from build123d import *

# Parameters (mm, degrees)
F1_DEPTH     = 63.5
F0_W         = 25.4
F0_H         = 19.05
F2_DEPTH     = 25.4
F3_DEPTH     = 7.9375
F5_R         = 5.08
F6_T         = 5.08
F6_T3_DEPTH  = 29.21
F6_T5_DEPTH  = 27.6225
F6_T7_DEPTH  = 73.66
F6_T9_DEPTH  = 27.6352
F6_T11_DEPTH = 27.6225
F6_T14_ANGLE = 84.6365269518
F6_T16_ANGLE = 180.000000001
F6_T18_ANGLE = 180.000000001
F6_T20_ANGLE = 84.6365269518


# Not quite as in the source:
# - a shell that OpenCascade refuses in one call is made with other operations: the cavity is built on its own and cut out


with BuildPart() as f1:
    # F0 (on Front) → F1 (new body, symmetric)
    with BuildSketch(Plane.XZ):
        Polygon((22.225, 9.525), (-41.275, 9.525), (-41.275, -9.525), (41.275, -9.525), (41.275, 9.525), align=None)
    extrude(amount=F1_DEPTH, both=True)

    # F0 (on Front) → F2 (join, symmetric)
    with BuildSketch(Plane.XZ):
        with BuildLine():
            Line((22.225, 27.0002), (22.225, 9.525))
            Line((22.225, 9.525), (41.275, 9.525))
            Line((41.275, 9.525), (41.275, 27.0002))
            ThreePointArc((41.275, 27.0002), (45.9246798487, 38.2255201513), (57.15, 42.8752))
            Line((57.15, 42.8752), (60.325, 42.8752))
            Line((60.325, 42.8752), (60.325, 61.9252))
            Line((60.325, 61.9252), (57.15, 61.9252))
            add(Edge.make_bspline(
                [(53.8854342407, 61.7722898912), (54.9842067368, 61.8365871986), (56.0728453275, 61.8876096574), (57.15, 61.9252)],
                knots=[108.5245810491, 108.5245810491, 108.5245810491, 108.5245810491, 111.5045361635, 111.5045361635, 111.5045361635, 111.5045361635], degree=3))
            ThreePointArc((53.8854342407, 61.7722898912), (31.3258777096, 50.5133948686), (22.225, 27.0002))
        make_face()
        with Locations((73.025, 52.4002)):
            Rectangle(F0_W, F0_H)
    extrude(amount=F2_DEPTH, both=True)

    # F0 (on Front) → F3 (join, symmetric)
    with BuildSketch(Plane.XZ):
        with BuildLine():
            add(Edge.make_bspline(
                [(-41.275, 9.525), (-39.5856284224, 39.4828766469), (13.870125209, 59.4306981306), (53.8854342407, 61.7722898912)],
                knots=[0, 0, 0, 0, 108.5245810491, 108.5245810491, 108.5245810491, 108.5245810491], degree=3))
            Line((-41.275, 9.525), (22.225, 9.525))
            Line((22.225, 9.525), (22.225, 27.0002))
            ThreePointArc((22.225, 27.0002), (31.3258777096, 50.5133948686), (53.8854342407, 61.7722898912))
        make_face()
    extrude(amount=F3_DEPTH, both=True)

    # F0 (on Front) → F4 (revolve)
    with BuildSketch(Plane.XZ):
        Polygon((85.725, 66.675), (85.725, 61.9252), (85.725, 42.8752), (85.725, 38.1), (111.125, 38.1), (111.125, 66.675), align=None)
    revolve(axis=Axis((85.725, 0, 52.3875), (0, 0, 1)))

    # F5
    f5_edges = [f1.edges().sort_by_distance(p)[0] for p in [
        (41.275, -63.5, 0),
        (-41.275, -63.5, 0),
        (41.275, 63.5, 0),
        (-41.275, 63.5, 0),
    ]]
    fillet(f5_edges, radius=F5_R)

    # F6: shell of thickness 5.08, made by hand


with BuildPart() as f6_core1:
    # F6_t2: copy of F1
    add(f1.part)

    # the walls: a layer under each face that stays
    f6_faces = [f6_core1.faces().sort_by_distance(p)[0] for p in [
        (0, 35.71875, 9.525),
        (41.275, 0, 8.7376),
        (32.8083333333, 25.4, 18.2583666667),
        (0, 63.5, 0),
        (22.225, 16.66875, 18.2626),
        (6.3052171204, 7.9375, 35.6486449456),
        (-41.275, 0, 0),
        (45.9246798487, 0, 38.2255201513),
        (32.8083333333, -25.4, 18.2583666667),
        (0, -35.71875, 9.525),
        (31.3258777096, 16.66875, 50.5133948686),
        (61.9125, 16.9333333333, 42.8752),
        (98.425, 21.9970452561, 42.8625),
        (61.9125, 16.9333333333, 61.9252),
        (55.5258238042, 12.7, 61.8587600574),
        (-8.0670094249, 3.96875, 46.0047517779),
        (-8.0670094249, -3.96875, 46.0047517779),
        (0, -63.5, 0),
        (31.3258777096, -16.66875, 50.5133948686),
        (22.225, -16.66875, 18.2626),
        (55.5258238042, -12.7, 61.8587600574),
        (6.3052171204, -7.9375, 35.6486449456),
        (85.725, 0, 66.675),
    ]]
    thicken(f6_faces, amount=-F6_T, mode=Mode.SUBTRACT)

    # F6_s4 → F6_t3 (cut)
    with BuildSketch(Plane.YZ.offset(17.145)):
        Polygon((25.4508, 9.5758), (25.4, 4.445), (20.32, 4.445), (20.32, 9.525), align=None)
        Polygon((-25.4508, 9.5758), (-20.32, 9.525), (-20.32, 4.445), (-25.4, 4.445), align=None)
    extrude(amount=F6_T3_DEPTH, mode=Mode.SUBTRACT)

    # F6_s6 → F6_t5 (cut)
    with BuildSketch(Plane.XZ.offset(-30.48)):
        Polygon((22.1742, 9.5758), (22.225, 4.445), (27.305, 4.445), (27.305, 9.525), align=None)
    extrude(amount=F6_T5_DEPTH, mode=Mode.SUBTRACT)

    # F6_s8 → F6_t7 (cut)
    with BuildSketch(Plane.YZ.offset(-46.355)):
        Polygon((7.9883, 9.5758), (7.9375, 4.445), (2.8575, 4.445), (2.8575, 9.525), align=None)
        Polygon((-7.9883, 9.5758), (-7.9375, 4.445), (-2.8575, 4.445), (-2.8575, 9.525), align=None)
    extrude(amount=F6_T7_DEPTH, mode=Mode.SUBTRACT)

    # F6_s10 → F6_t9 (cut)
    with BuildSketch(Plane.XY.offset(4.445)):
        Polygon((22.1742, 7.9883), (27.305, 7.9375), (27.305, 2.8575), (22.225, 2.8575), align=None)
        Polygon((22.1742, -7.9883), (27.305, -7.9375), (27.305, -2.8575), (22.225, -2.8575), align=None)
    extrude(amount=F6_T9_DEPTH, mode=Mode.SUBTRACT)

    # F6_s12 → F6_t11 (cut)
    with BuildSketch(Plane.XZ.offset(2.8575)):
        Polygon((22.1742, 9.5758), (22.225, 4.445), (27.305, 4.445), (27.305, 9.525), align=None)
    extrude(amount=F6_T11_DEPTH, mode=Mode.SUBTRACT)

    # F6_s13 → F6_t14 (revolve, cut)
    with BuildSketch(Plane.XY.offset(27.0002)):
        Polygon((22.1742, 7.9883), (22.225, 2.8575), (27.305, 2.8575), (27.305, 7.9375), align=None)
    revolve(axis=Axis((57.15, 7.9375, 27.0002), (0, 1, 0)), revolution_arc=F6_T14_ANGLE, mode=Mode.SUBTRACT)

    # F6_s15 → F6_t16 (revolve, cut)
    with BuildSketch(Plane.YZ.offset(85.725)):
        Polygon((25.4508, 42.8244), (25.4, 47.9552), (20.32, 47.9552), (20.32, 42.8752), align=None)
    revolve(axis=Axis((85.725, 0, 42.8752), (0, 0, 1)), revolution_arc=F6_T16_ANGLE, mode=Mode.SUBTRACT)

    # F6_s17 → F6_t18 (revolve, cut)
    with BuildSketch(Plane.YZ.offset(85.725)):
        Polygon((25.4508, 61.976), (20.32, 61.9252), (20.32, 56.8452), (25.4, 56.8452), align=None)
    revolve(axis=Axis((85.725, 0, 61.9252), (0, 0, 1)), revolution_arc=F6_T18_ANGLE, mode=Mode.SUBTRACT)

    # F6_s19 → F6_t20 (revolve, cut)
    with BuildSketch(Plane.XY.offset(27.0002)):
        Polygon((22.1742, -7.9883), (27.305, -7.9375), (27.305, -2.8575), (22.225, -2.8575), align=None)
    revolve(axis=Axis((57.15, -7.9375, 27.0002), (0, 1, 0)), revolution_arc=F6_T20_ANGLE, mode=Mode.SUBTRACT)


with BuildPart() as f1_1:
    add(f1.part)

    # what is left inside the walls is the cavity
    f6_cavity = [f6_core1.part.solids().sort_by_distance(p)[0] for p in [
        (0, 19.473333, -9.4742),
    ]]
    add(f6_cavity, mode=Mode.SUBTRACT)


solid = f1_1.part
Here's how the part is built. I have some questions about the finished solid (model axes, mm). A direction names the side the tool comes from. Give positions to 0.01 mm unless a question says otherwise; leave off trailing zeros. Order: outer loops, then holes, each group sorted by start corner. A loop starts at its lowest first (then second) coordinate and runs counter-clockwise, first axis right, second up. Notation, with made-up numbers: M -38.5,65.25 L 19.5,65.25 A16 cw 19.5,88.25 Z; hole C 37,51 d1. An arc over 180 degrees is marked long. Answer as a JSON object with one key per item and string values. Group by question number.
1) Please list where these lines run through material, in increasing order: L1, parallel to Y at x = 36, z = 46; L2, parallel to Y at x = 10, z = -5.5; L3, parallel to X at y = 0, z = 44 (3 decimals). Write a range as [from, to].
2) On a 3-axis mill with a long thin cutter (end or side, diameter ignored), from which of +Z, -Z, +X, -X, +Y, -Y can I reach the whole of each face in a straight line? I mean faces 5 (the flat face through (60, -2, 61.925)), 6 (the flat face through (27.305, -12, 16)), 7 (the flat face through (65, 0, 56.845)). Say none if no direction works.
3) Suppose I cut it at A-A, the plane z = 6.5. Write out the boundary of the cut face in (x, y) (1 decimal), plus the area to 3 significant figures.
4) We'd pull the mould along X, two halves only. Please class faces 1 (the cylindrical face through (39.8, -62, 0.1)), 2 (the flat face through (-41.275, -1, 0)), 3 (the flat face through (47.7, 20.32, 46.3)), 4 (the flat face through (-2, 2.858, 24)): pulls with the +X half, pulls with the -X half, needs draft (parallel to the pull), parting line crosses it, or undercut.
5) I'm going to push flat-ended pins straight in: pin 1 Ø8.5 at (y, z) = (14, 12) entering from +X (3 decimals); pin 2 Ø8 at (x, z) = (25.5, 26.5) entering from +Y; pin 3 Ø15 at (x, y) = (73.5, 9) entering from -Z. Where does each tip first touch, or does it pass through?
6) Suppose I cut it at B-B, the plane y = 55. Write out the boundary of the cut face in (x, z) (3 decimals), plus the area to 3 significant figures.
Results found:
{
 "1": {"L1": "[-25.4, -20.32], [20.32, 25.4]", "L2": "[-63.5, -58.42], [58.42, 63.5]", "L3": "[-12.006, -0.213], [44.898, 65.405], [106.045, 111.125]"},
 "2": {"face 5": "+Z, -X", "face 6": "-Z", "face 7": "none"},
 "3": {"outline": "M -41.3,-58.4 A5.1 ccw -36.2,-63.5 L 36.2,-63.5 A5.1 ccw 41.3,-58.4 L 41.3,58.4 A5.1 ccw 36.2,63.5 L -36.2,63.5 A5.1 ccw -41.3,58.4 Z; hole M -36.2,-2.9 L 27.3,-2.9 L 27.3,-20.3 L 36.2,-20.3 L 36.2,20.3 L 27.3,20.3 L 27.3,2.9 L -36.2,2.9 Z", "area": "9,740 mm²"},
 "4": {"face 1": "pulls with the +X half", "face 2": "pulls with the -X half", "face 3": "undercut", "face 4": "undercut"},
 "5": {"pin 1": "x = 41.275", "pin 2": "y = 25.4", "pin 3": "z = 38.1"},
 "6": {"outline": "M -41.275,-9.525 L -36.195,-9.525 L -36.195,4.445 L 36.195,4.445 L 36.195,-9.525 L 41.275,-9.525 L 41.275,9.525 L -41.275,9.525 Z", "area": "561 mm²"}
}
